Part print with two shaded views. Sizes in mm from the minimum x, y, z corner. A direction names the side the tool comes from. Coordinates: 2 decimals unless noted, no trailing zeros. Order: outer loops, then holes, each group sorted by start corner. A loop starts at its lowest first (then second) coordinate and runs counter-clockwise, first axis right, second up. Notation, with made-up numbers: (78, 49) - (101, 49) arc R17 cw to (101, 82) - close; hole circle Ø10 at (86.5, 69). An arc over 180 degrees is marked (long way). Return JSON: item names as keys, results as strings.
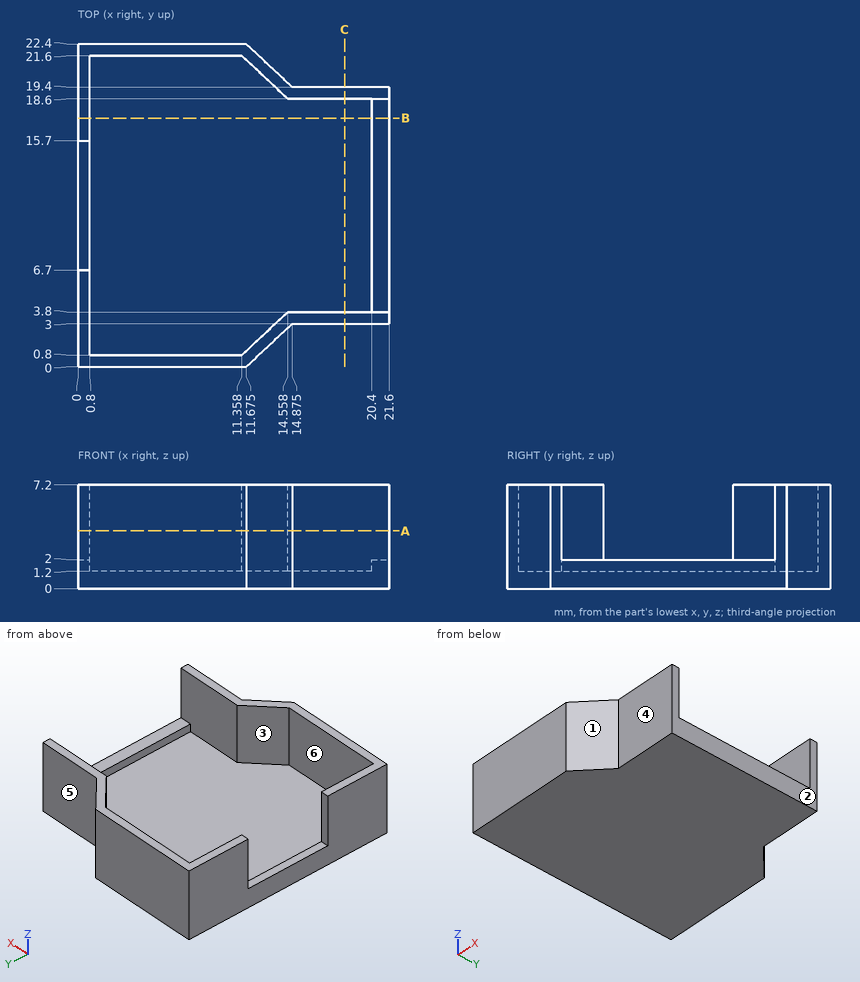
Item 1: Band-saw the part on A-A, the plane z = 4. List the corners of the cut face in (x, y) (1 decimal).
Findings below:
{"outline": "(0, 0) - (11.7, 0) - (14.9, 3) - (21.6, 3) - (21.6, 3.8) - (14.6, 3.8) - (11.4, 0.8) - (0.8, 0.8) - (0.8, 6.7) - (0, 6.7) - close; (0, 15.7) - (0.8, 15.7) - (0.8, 21.6) - (11.4, 21.6) - (14.6, 18.6) - (21.6, 18.6) - (21.6, 19.4) - (14.9, 19.4) - (11.7, 22.4) - (0, 22.4) - close"}
Item 2: Wall check: L1, parallel to Y at x = 16, z = 5.75; L2, parallel to Y at x = 1.75, z = 3.25; L3, parallel to X at y = 12.5, z = 1.25. Give the ranges that are in metal, low to high. Write a range as [from, to].
Findings below:
{"L1": "y = [3, 3.8], [18.6, 19.4]", "L2": "y = [0, 0.8], [21.6, 22.4]", "L3": "x = [0, 0.8], [20.4, 21.6]"}
Item 3: Mould opens along Y. For the marked faces 1, 2 and 3 say: released by +Y, released by -Y, zero draft, split by the parting line, or undercut.
Findings below:
{"face 1": "released by -Y", "face 2": "zero draft", "face 3": "undercut"}
Item 4: Drop flat-ended pins along their axis: P1, Ø1, axis at x = 4, y = 13.5, coming from the -Z side; P2, Ø1.8, axis at x = 18.5, z = 3, coming from the +Y side; P3, Ø6, axis at x = 14.5, y = 15, coming from the +Z side; P4, Ø0.9, axis at x = 0.5, y = 12.5, coming from the +Z side. Give the stop position or say it passes through.
Findings below:
{"P1": "stops at z = 0", "P2": "stops at y = 19.4", "P3": "stops at z = 1.2", "P4": "stops at z = 2"}
Item 5: Band-saw the part on B-B, the plane y = 17.25. List the corners of the cut face in (x, z).
Findings below:
{"outline": "(0, 0) - (21.6, 0) - (21.6, 2) - (20.4, 2) - (20.4, 1.2) - (0.8, 1.2) - (0.8, 7.2) - (0, 7.2) - close"}
Item 6: Which spindle directions (+Z, -Z, +X, -X, +Y, -Y) get a long thin tool onto all of the face, cutting with end or side? Do the marked faces 4, 5 and 6. Say none if no direction does.
Findings below:
{"face 4": "+Z, -Z, +X, -Y", "face 5": "+Z, -Z, +X, +Y", "face 6": "+Z"}
Item 7: Band-saw the part on C-C, the plane x = 18.5. List the corners of the cut face in (y, z).
Findings below:
{"outline": "(3, 0) - (19.4, 0) - (19.4, 7.2) - (18.6, 7.2) - (18.6, 1.2) - (3.8, 1.2) - (3.8, 7.2) - (3, 7.2) - close"}
